Work out the finished part from the listing and answer in its coordinate system (mm). Face numbers are marked on the shaded views. A direction names the side the tool comes from. Coordinates: 2 decimals unless noted, no trailing zeros. Order: outer loops, then holes, each group sorted by start corner. A loop starts at its lowest first (then second) coordinate and runs counter-clockwise, first axis right, second up.
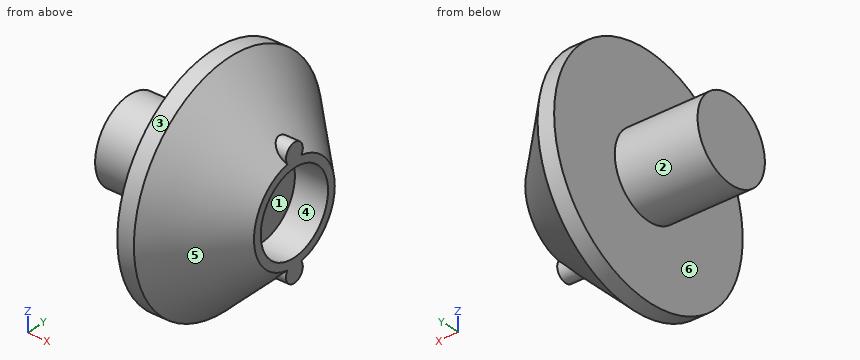
```python
from build123d import *

# Parameters (mm, degrees)
F0_R     = 17.78
F0_R_2   = 1.5875
F0_R_3   = 6.35
F1_DEPTH = 12.7
F3_DEPTH = 7.62
F4_DEPTH = 12.7
F5_DEPTH = 12.7


# Not quite as in the source:
# - a fillet or chamfer that OpenCascade refuses, or shapes differently, is made with other operations: its cross-section is extruded or revolved along the edge and cut away or added


with BuildPart() as f1:
    # F0 (on Right) → F1 (new body)
    with BuildSketch(Plane.YZ):
        Circle(F0_R)
        with Locations((0, -8.382)):
            Circle(F0_R_2, mode=Mode.SUBTRACT)
        Circle(F0_R_3, mode=Mode.SUBTRACT)
        with Locations((0, 8.382)):
            Circle(F0_R_2, mode=Mode.SUBTRACT)
    extrude(amount=F1_DEPTH)

    # F2: chamfer of 10.16 on 1 edges, made by hand

    # F2_s1 → F2_t2 (revolve, cut)
    with BuildSketch(Plane.XY):
        Polygon((2.54, 17.78), (12.7, 7.62), (12.7, 17.78), align=None)
    revolve(axis=Axis((12.7, 0, 0), (1, 0, 0)), mode=Mode.SUBTRACT)

    # F0 (on Right) → F3 (join)
    with BuildSketch(Plane.YZ):
        Circle(F0_R_3)
    extrude(amount=F3_DEPTH)

    # F0 (on Right) → F4 (join)
    with BuildSketch(Plane.YZ):
        with Locations((0, 8.382)):
            Circle(F0_R_2)
        with Locations((0, -8.382)):
            Circle(F0_R_2)
    extrude(amount=F4_DEPTH)

    # F0 (on Right) → F5 (join)
    with BuildSketch(Plane.YZ):
        Circle(F0_R_3)
    extrude(amount=-F5_DEPTH)


solid = f1.part
```
1. The mould has two halves that part along Y. Classify the marked faces 4, 5 and 6: released by +Y, released by -Y, zero draft, split by the parting line, or undercut.
2. The part is cut by section C-C (x = 4.5). Determine the outline of the cut face in (y, z), plus the area to 3 significant figures.
3. The part is cut by section A-A (z = 0). Determine the outline of the cut face in (x, y), plus the area to 3 significant figures.
4. The part is cut by section B-B (y = 0). Determine the outline of the cut face in (x, z).
5. The part is cut by section D-D (x = -4). Determine the outline of the cut face in (y, z).
6. Consider probe 1 along Z at (x, y) = (10.8, 0); probe 2 along X at (y, z) = (6, 4); probe 3 along Z at (x, y) = (8.9, 0). Determine where each line is inside the solid, lowest interval first.
7. Flat-ended cylindrical pins translate along their axes: pin 1 (12 mm diameter, centred on x = 4.5, y = 0.5, fed in from +Z); pin 2 (12 mm diameter, centred on x = 5, y = -7.5, fed in from +Z); pin 3 (8 mm diameter, centred on x = 3.5, z = -8.5, fed in from -Y); pin 4 (2 mm diameter, centred on x = 5, y = -7, fed in from -Z). Find the tip coordinate at first contact, or state that the pin passes through.
8. For the marked faces 1, 2 and 3, determine the directions among +Z, -Z, +X, -X, +Y, -Y from which every point of the face is accessible in a straight line to the end or side of a thin tool.
Worked out:
1. face 4: undercut
1. face 5: split by the parting line
1. face 6: zero draft
2. outline: circle Ø31.64 at (0, 0)
2. area: 786 mm2
3. outline: (-12.7, -6.35) - (0, -6.35) - (0, -17.78) - (2.54, -17.78) - (12.7, -7.62) - (12.7, -6.35) - (7.62, -6.35) - (7.62, 6.35) - (12.7, 6.35) - (12.7, 7.62) - (2.54, 17.78) - (0, 17.78) - (0, 6.35) - (-12.7, 6.35) - close
3. area: 445 mm2
4. outline: (-12.7, -6.35) - (0, -6.35) - (0, -17.78) - (2.54, -17.78) - (10.35, -9.97) - (12.7, -9.97) - (12.7, -6.35) - (7.62, -6.35) - (7.62, 6.35) - (12.7, 6.35) - (12.7, 9.97) - (10.35, 9.97) - (2.54, 17.78) - (0, 17.78) - (0, 6.35) - (-12.7, 6.35) - close
5. outline: circle Ø12.7 at (0, 0)
6. probe 1: z = -9.97 to -6.35, 6.35 to 9.97
6. probe 2: x = 0 to 12.7
6. probe 3: z = -11.42 to -6.35, 6.35 to 11.42
7. pin 1: stops at z = 17.78
7. pin 2: stops at z = 17.66
7. pin 3: stops at y = -17.17
7. pin 4: stops at z = -14.83
8. face 1: +X
8. face 2: -X
8. face 3: +X, -X
